```python
from build123d import *

# Parameters (mm, degrees)
F0_W     = 141.7553946376
F0_H     = 141.903989017
F1_DEPTH = 76.2
F2_R     = 35.6206675953
F3_DEPTH = 152.4
F5_DEPTH = 0.508
F6_R     = 2.3752413704
F7_DEPTH = 7.62


with BuildPart() as f1:
    # F0 (on Front) → F1 (new body)
    with BuildSketch(Plane.XZ):
        with Locations((0.6661005318, -0.6118379533)):
            Rectangle(F0_W, F0_H)
    extrude(amount=F1_DEPTH)

    # F2 (on face) → F3 (cut)
    with BuildSketch(Plane(origin=(-70.211596787, 0, 0), x_dir=(0, -1, 0), z_dir=(-1, 0, 0))):
        with Locations((38.8970784843, 0)):
            Circle(F2_R)
    extrude(amount=-F3_DEPTH, mode=Mode.SUBTRACT)

    # F4 (on face) → F5 (join)
    with BuildSketch(Plane(origin=(0, 0, -71.5638324618), x_dir=(1, 0, 0), z_dir=(0, 0, -1))):
        with BuildLine():
            add(Edge.make_bspline(
                [(-54.6526201069, 43.9366996288), (-54.6526201069, 27.8657274233), (27.3263100535, 35.901213526), (109.3052402139, 43.9366996288), (27.3263100535, 51.9721857316), (-54.6526201069, 60.0076718344), (-54.6526201069, 43.9366996288)],
                knots=[0, 0, 0, 2.0943951024, 2.0943951024, 4.1887902048, 4.1887902048, 6.2831853072, 6.2831853072, 6.2831853072], degree=2, weights=[1, 0.5, 1, 0.5, 1, 0.5, 1]))
        make_face()
    extrude(amount=F5_DEPTH)

    # F6 (on face) → F7 (cut)
    with BuildSketch(Plane(origin=(0, 0, -71.5638324618), x_dir=(1, 0, 0), z_dir=(0, 0, -1))):
        with Locations((-64.7707954049, 72.0797255635)):
            Circle(F6_R)
    extrude(amount=-F7_DEPTH, mode=Mode.SUBTRACT)


solid = f1.part
```
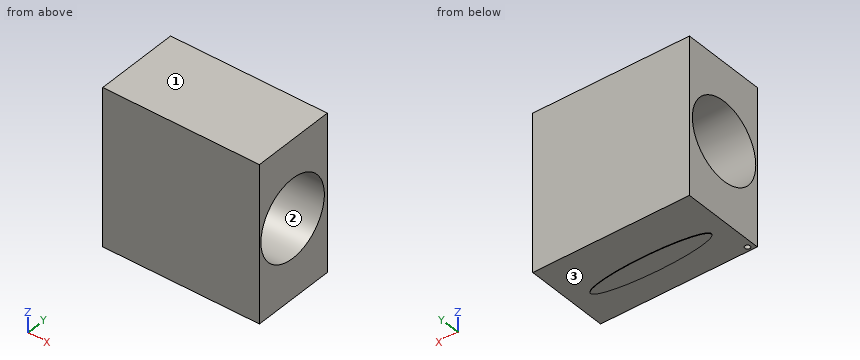
Can you work these out from the model? Positions are in its coordinate system, mm. Face numbers are marked on the shaded views. Coordinates: 2 decimals unless noted, no trailing zeros. Loops run counter-clockwise (first coordinate to the right, second up) from the corner with the lowest first, then second, coordinate; pieces in that order, holes last.
1) Imagine slicing it at B-B on y = -26. List the corners of the cut face in (x, z) for me, plus the area to 3 significant figures.
2) For pin 1 (2.5 mm diameter, centred on x = -66, y = -72, fed in from -Z), with a flat end and sliding along its axis, tell me the tip position at first contact or that it passes through.
3) Imagine slicing it at A-A on z = 0. List the corners of the cut face in (x, y) for me, plus the area to 3 significant figures.
4) Thinking about a two-plate mould opening in Z: for the marked faces 1, 2 and 3, which applies, pulls with the +Z half, pulls with the -Z half, needs draft (parallel to the pull), parting line crosses it, or undercut?
5) I need wall thicknesses on probe 1 along Z at (x, y) = (15, -25.5); probe 2 along Z at (x, y) = (-24, -36); probe 3 along Y at (x, z) = (-60, 7.5). Which ranges of each line are inside material? Lowest first, please.
Completed:
1. outline: (-70.21, -71.56) - (71.54, -71.56) - (71.54, -33.2) - (-70.21, -33.2) - close; (-70.21, 33.2) - (71.54, 33.2) - (71.54, 70.34) - (-70.21, 70.34) - close
1. area: 10,700 mm2
2. pin 1: stops at z = -71.56
3. outline: (-70.21, -76.2) - (71.54, -76.2) - (71.54, -74.52) - (-70.21, -74.52) - close; (-70.21, -3.28) - (71.54, -3.28) - (71.54, 0) - (-70.21, 0) - close
3. area: 703 mm2
4. face 1: pulls with the +Z half
4. face 2: undercut
4. face 3: pulls with the -Z half
5. probe 1: z = -71.56 to -33.01, 33.01 to 70.34
5. probe 2: z = -72.07 to -35.5, 35.5 to 70.34
5. probe 3: y = -76.2 to -73.72, -4.07 to 0
